Design review of the part shown in the three views and the two pictorial views. Dimensions are in mm from the part's minimum x, y and z. Round coordinates to 2 decimals unless told otherwise and drop trailing zeros. Loops run counter-clockwise (first coordinate to the right, second up) from the corner with the lowest first, then second, coordinate; pieces in that order, holes last.
1. Draft analysis for pull direction X (two halves, no side actions). For the marked faces 1, 2 and 3, state which applies: released by +X, released by -X, zero draft, split by the parting line, or undercut.
2. To check wall thickness, follow line 1 along Y through (x, z) = (10.5, 0.7); line 2 along Y through (x, z) = (14, 0.85); line 3 along Y through (x, z) = (18, 1.4). State the ranges of each line that lie inside material, in increasing order.
3. Consider section C-C on z = 1.3. State how many separate pieces and enclosed holes the cut face has, then the cut area to 3 significant figures.
4. Consider section B-B on y = 11.5. State the section outline as (x, z) points.
5. Clearance check with flat-ended pins moving along their axes: pin 1 Ø1.4 at (x, y) = (3, 7) entering from +Z; pin 2 Ø1 at (x, z) = (7.5, 0.5) entering from -Y. State where each tip first meets the part, or that it passes through.
6. Consider section A-A on x = 10.5. State the section outline as (y, z) points.
7. Consider section D-D on x = 7. State the section outline as (y, z) points.
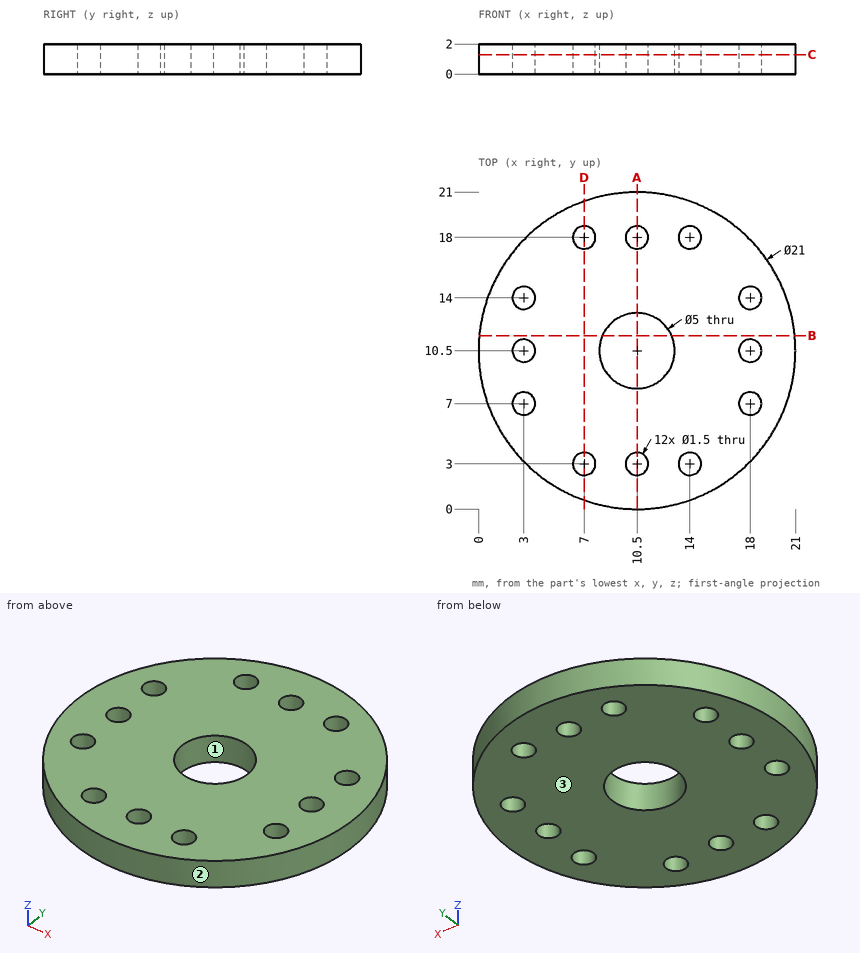
Resolved:
1. face 1: undercut
1. face 2: split by the parting line
1. face 3: zero draft
2. line 1: y = 0 to 2.25, 3.75 to 8, 13 to 17.25, 18.75 to 21
2. line 2: y = 0.6 to 2.25, 3.75 to 17.25, 18.75 to 20.4
2. line 3: y = 3.15 to 6.25, 7.75 to 9.75, 11.25 to 13.25, 14.75 to 17.85
3. separate pieces: 1
3. enclosed holes: 13
3. area: 306 mm2
4. outline: (0.05, 0) - (8.21, 0) - (8.21, 2) - (0.05, 2) - close; (12.79, 0) - (20.95, 0) - (20.95, 2) - (12.79, 2) - close
5. pin 1: passes through
5. pin 2: stops at y = 0.3
6. outline: (0, 0) - (2.25, 0) - (2.25, 2) - (0, 2) - close; (3.75, 0) - (8, 0) - (8, 2) - (3.75, 2) - close; (13, 0) - (17.25, 0) - (17.25, 2) - (13, 2) - close; (18.75, 0) - (21, 0) - (21, 2) - (18.75, 2) - close
7. outline: (0.6, 0) - (2.25, 0) - (2.25, 2) - (0.6, 2) - close; (3.75, 0) - (17.25, 0) - (17.25, 2) - (3.75, 2) - close; (18.75, 0) - (20.4, 0) - (20.4, 2) - (18.75, 2) - close
